```python
from build123d import *

# Parameters (mm, degrees)
SKETCH2_R           = 6.35
BOSS_EXTRUDE1_DEPTH = 40
FILLET1_R           = 10
SKETCH5_R           = 4


with BuildPart() as part:
    # Sketch2 → Boss-Extrude1 (new body)
    with BuildSketch(Plane(origin=(0, 0, 0), x_dir=(1, 0, 0), z_dir=(0, 1, 0))):
        with Locations(Location((0, 0, 0), (0, 0, 270))):
            Circle(SKETCH2_R)
    extrude(amount=BOSS_EXTRUDE1_DEPTH)

    # Sketch4 → Revolve1 (revolve)
    with BuildSketch(Plane.XY, mode=Mode.PRIVATE) as revolve1_sk:
        with BuildLine():
            Line((0, 40), (34.903897247, 40))
            ThreePointArc((34.903897247, 40), (31.810988232, 46.594188763), (30.75, 53.8))
            Line((30.75, 53.8), (30.75, 88.8))
            Line((30.75, 88.8), (14.55, 105))
            Line((14.55, 105), (0, 105))
            Line((0, 105), (0, 40))
        make_face()
    revolve(revolve1_sk.sketch.rotate(Axis((0, 40, 0), (0, 1, 0)), 90), axis=Axis((0, 40, 0), (0, 1, 0)))

    # Fillet1
    fillet1_edges = [part.edges().sort_by_distance(p)[0] for p in [
        (0, 40, -6.35),
    ]]
    fillet(fillet1_edges, radius=FILLET1_R)

    # Sketch5 → Cut-Loft1 section 0
    with BuildSketch(Plane(origin=(0, 105, 0), x_dir=(1, 0, 0), z_dir=(0, 1, 0)), mode=Mode.PRIVATE) as cut_loft1_s0:
        Circle(SKETCH5_R)
    loft([Vertex(0, 95, 0), cut_loft1_s0.sketch], mode=Mode.SUBTRACT)


solid = part.part
```
Input: part model. Units: mm. Frame: model coordinates. A direction names the side the tool comes from. Coordinates: 2 decimals unless noted, no trailing zeros. Loops run counter-clockwise (first coordinate to the right, second up) from the corner with the lowest first, then second, coordinate; pieces in that order, holes last.
Q1. Section A-A, the plane y = 98.5. Return the cut outline in (x, z).
Results are:
outline: circle Ø42.1 at (0, 0); hole circle Ø2.8 at (0, 0)
Q2. Section B-B, the plane y = 84. Return the cut outline in (x, z), and give its area (3 significant figures).
Results are:
outline: circle Ø61.5 at (0, 0)
area: 2,970 mm2
Q3. Set-up query: faces 4 (the flat face through (0, 0, 0)), 5 (the cylindrical face through (-3.86, 14.79, -5.04)), 6 (the cylindrical face through (-30.49, 71.54, 4)). Return all of +Z, -Z, +X, -X, +Y, -Y with unobstructed straight access to the full face (end or side cutting, diameter ignored); none if empty.
Results are:
face 4: +Z, -Z, +X, -X, -Y
face 5: -Y
face 6: +Y
Q4. Section C-C, the plane y = 27. Return the cut outline in (x, z).
Results are:
outline: circle Ø12.7 at (0, 0)
Q5. Line query: line 1 along Z through (x, y) = (1, 64.5); line 2 along X through (y, z) = (65, 0); line 3 along X through (y, z) = (48, 21). Output: solid intervals per line, ascending.
Results are:
line 1: z = -30.73 to 30.73
line 2: x = -30.75 to 30.75
line 3: x = -23.39 to 23.39
Q6. Contact query for flat-ended pins moving along their axis: pin 1 (3 mm diameter, centred on x = -21.5, y = 56.5, fed in from -Z); pin 2 (8 mm diameter, centred on x = 11, y = 58, fed in from -Z); pin 3 (12 mm diameter, centred on x = 23, y = 86.5, fed in from -Z). Output: stop coordinate, or through.
Results are:
pin 1: stops at z = -23.36
pin 2: stops at z = -29.94
pin 3: stops at z = -25.62
Q7. Mould query, pull axis Z, two halves, no side actions, for faces 1 (the flat face through (7, 40, 15)), 2 (the conical face through (-4.61, 104.21, -14.63)), 3 (the conical face through (-0.343, 98.959, 1.546)). Classes: +Z half, -Z half, draft (parallel to the pull), parting line (faces both ways), or undercut.
Results are:
face 1: draft
face 2: parting line
face 3: undercut
